Check sheet for the modelled part. Datum: model origin and axes. Units: mm. A direction names the side the tool comes from. Coordinates: 2 decimals unless noted, no trailing zeros. Write each loop counter-clockwise with the first axis right and the second up, starting at its lowest first coordinate (ties: lowest second). Pieces come first, ordered by that corner, then holes. Notation, with made-up numbers: M 72.5,6 L 82.5,6 A23 cw 82.5,18 Z; hole C -33.5,49.25 d4. An arc over 180 degrees is marked long. Answer as CSV lines item,"result". Start each with the question number.
1) Material ranges on L1, parallel to Y at x = 0, z = 1.1; L2, parallel to X at y = 29.5, z = 0.3; L3, parallel to X at y = -2.5, z = 4.75, recorded low to high. Write a range as [from, to].
2) Draft check along Y on faces 1 (the flat face through (-4.5, -43, 1)), 2 (the flat face through (-38, -62, 3)), 3 (the flat face through (68.5, 1, 4)). Enter one of: +Y half, -Y half, draft (parallel to the pull), parting line (faces both ways), or undercut.
3) Access from +Z, -Z, +X, -X, +Y, -Y to the whole of each face (thin tool, end or side, straight path). Record for faces 4 (the flat face through (36, 60, 4)), 5 (the flat face through (20.71, 42.57, 0.99)).
4) Go/stop test with a flat-tipped pin: pin 1 Ø3 at (x, y) = (0, 8) entering from +Z. Record where the tip stops, or that it passes through.
5) Section check A-A (y = 1). Record the cut outline in (x, z).
6) Section check B-B (y = 47.5). State how many separate pieces and enclosed holes the cut face has, and give its area (3 significant figures).
from build123d import *

# Parameters (mm, degrees)
F0_W     = 64
F0_H     = 120
F2_DEPTH = 2
F3_DEPTH = 6
F4_W     = 6
F4_H     = 12
F4_W_2   = 12
F4_H_2   = 6
F5_DEPTH = 2
F7_DEPTH = 2
F8_W     = 9
F8_H     = 40
F8_R     = 1
F9_DEPTH = 2
F10_R    = 1.99999
F11_R    = 1.99999


# Not quite as in the source:
# - a fillet or chamfer is up to 0.001 mm smaller than in the source, because OpenCascade refuses the exact size


with BuildPart() as f2:
    # F0 (on Top) → F2 (new body)
    with BuildSketch(Plane.XY):
        with Locations((-36.5, 0)):
            Rectangle(F0_W, F0_H)
    extrude(amount=F2_DEPTH)

    # F1 (on Top) → F3 (join)
    with BuildSketch(Plane.XY):
        Polygon((-4.5, 60), (-4.5, 62), (-70.5, 62), (-70.5, -62), (-4.5, -62), (-4.5, -60), (-68.5, -60), (-68.5, 60), align=None)
    extrude(amount=F3_DEPTH)

    # F4 (on face) → F5 (join)
    with BuildSketch(Plane.XY.offset(6)):
        with Locations((-67.5, 46)):
            Rectangle(F4_W, F4_H)
        with Locations((-28.5, 59)):
            Rectangle(F4_W_2, F4_H_2)
        with Locations((-67.5, 22)):
            Rectangle(F4_W, F4_H)
        with Locations((-28.5, -59)):
            Rectangle(F4_W_2, F4_H_2)
        with Locations((-67.5, -22)):
            Rectangle(F4_W, F4_H)
        with Locations((-67.5, -46)):
            Rectangle(F4_W, F4_H)
    extrude(amount=-F5_DEPTH)


with BuildPart() as f2b:
    # F0 (on Top) → F2, piece 2 (new body)
    with BuildSketch(Plane.XY):
        with Locations((36.5, 0)):
            Rectangle(F0_W, F0_H)
    extrude(amount=F2_DEPTH)

    # F1 (on Top) → F3, piece 2 (join)
    with BuildSketch(Plane.XY):
        Polygon((70.5, -62), (70.5, 62), (4.5, 62), (4.5, 60), (68.5, 60), (68.5, -60), (4.5, -60), (4.5, -62), align=None)
    extrude(amount=F3_DEPTH)

    # F4 (on face) → F5, piece 2 (join)
    with BuildSketch(Plane.XY.offset(6)):
        with Locations((67.5, 46)):
            Rectangle(F4_W, F4_H)
        with Locations((67.5, -22)):
            Rectangle(F4_W, F4_H)
        with Locations((67.5, -46)):
            Rectangle(F4_W, F4_H)
        with Locations((28.5, 59)):
            Rectangle(F4_W_2, F4_H_2)
        with Locations((67.5, 22)):
            Rectangle(F4_W, F4_H)
        with Locations((28.5, -59)):
            Rectangle(F4_W_2, F4_H_2)
    extrude(amount=-F5_DEPTH)


with BuildPart() as f7_tool:
    # F6 (on face) → F7 (new body)
    with BuildSketch(Plane(origin=(0, 0, 0), x_dir=(1, 0, 0), z_dir=(0, 0, -1))):
        Polygon((-9.5378331968, 57.0000003456), (-63.1068291486, 57.0000003456), (-36.4934644097, 32.0499709028), align=None)
        Polygon((-7.5, 4.8685980187), (-7.5, 54.7983564456), (-34.2993455202, 29.9929844439), align=None)
        Polygon((-9.8931712199, 3), (-36.5065294908, 27.9500233789), (-63.4621541524, 3), align=None)
        Polygon((-65.4999873492, 5.2016438999), (-38.7006483802, 30.0070098378), (-65.5, 55.1314019813), align=None)
        Polygon((-63.4621541524, -3), (-36.5065294908, -27.9500233789), (-9.8931712199, -3), align=None)
        Polygon((-7.5, -4.8685980187), (-34.2993455202, -29.9929844439), (-7.5, -54.7983564456), align=None)
        Polygon((-9.5378331968, -57.0000003456), (-36.4934644097, -32.0499709028), (-63.1068291486, -57.0000003456), align=None)
        Polygon((-65.5, -55.1314019813), (-38.7006483802, -30.0070098378), (-65.4999873492, -5.2016438999), align=None)
        Polygon((7.5, -54.7983564456), (34.2993455202, -29.9929844439), (7.5, -4.8685980187), align=None)
        Polygon((63.1068291486, -57.0000003456), (36.4934644097, -32.0499709028), (9.5378331968, -57.0000003456), align=None)
        Polygon((65.5, -55.1314019813), (65.4999873492, -5.2016438999), (38.7006483802, -30.0070098378), align=None)
        Polygon((36.5065294908, -27.9500233789), (63.4621541524, -3), (9.8931712199, -3), align=None)
        Polygon((63.4621541524, 3), (36.5065294908, 27.9500233789), (9.8931712199, 3), align=None)
        Polygon((7.5, 4.8685980187), (34.2993455202, 29.9929844439), (7.5, 54.7983564456), align=None)
        Polygon((9.5378331968, 57.0000003456), (36.4934644097, 32.0499709028), (63.1068291486, 57.0000003456), align=None)
        Polygon((65.5, 55.1314019813), (38.7006483802, 30.0070098378), (65.4999873492, 5.2016438999), align=None)
    extrude(amount=-F7_DEPTH)


with BuildPart() as f2_1:
    add(f2.part)

    # F7: cut by f7_tool
    add(f7_tool.part, mode=Mode.SUBTRACT)



with BuildPart() as f2b_1:
    add(f2b.part)

    # F7: cut by f7_tool
    add(f7_tool.part, mode=Mode.SUBTRACT)


with BuildPart() as f2_2:
    add(f2_1.part)

    add(f2b_1.part)  # F9 merges F2b
    # F8 (on face) → F9 (join)
    with BuildSketch(Plane(origin=(0, 0, 0), x_dir=(1, 0, 0), z_dir=(0, 0, -1))):
        Rectangle(F8_W, F8_H)
        with Locations((0, -8)):
            Circle(F8_R, mode=Mode.SUBTRACT)
        with Locations((0, 8)):
            Circle(F8_R, mode=Mode.SUBTRACT)
    extrude(amount=-F9_DEPTH)

    # F10 (radius 2 in the source; OpenCascade refuses exactly that, so slightly less here)
    f10_edges = [f2_2.edges().sort_by_distance(p)[0] for p in [
        (28.5, -56, 4),
        (-28.5, -56, 4),
        (64.5, -46, 4),
        (64.5, -22, 4),
        (-64.5, -46, 4),
        (-64.5, -22, 4),
        (64.5, 22, 4),
        (64.5, 46, 4),
        (-28.5, 56, 4),
        (28.5, 56, 4),
        (-64.5, 22, 4),
        (-64.5, 46, 4),
    ]]
    fillet(f10_edges, radius=F10_R)

    # F11 (radius 2 in the source; OpenCascade refuses exactly that, so slightly less here)
    f11_edges = [f2_2.edges().sort_by_distance(p)[0] for p in [
        (28.5, -60, 4),
        (-28.5, -60, 4),
        (-68.5, -46, 4),
        (-68.5, -22, 4),
        (68.5, -46, 4),
        (68.5, -22, 4),
        (68.5, 46, 4),
        (68.5, 22, 4),
        (28.5, 60, 4),
        (-28.5, 60, 4),
        (-68.5, 22, 4),
        (-68.5, 46, 4),
    ]]
    fillet(f11_edges, radius=F11_R)


solid = f2_2.part
Results found:
1,L1,"y = [-20, -9], [-7, 7], [9, 20]"
1,L2,"x = [-70.5, -65.5], [-39.25, -33.77], [-7.5, -4.5], [4.5, 7.5], [33.77, 39.25], [65.5, 70.5]"
1,L3,"x = [-70.5, -68.5], [68.5, 70.5]"
2,face 1,"draft"
2,face 2,"-Y half"
2,face 3,"undercut"
3,face 4,"+Z"
3,face 5,"+Z, -Z"
4,pin 1,"stops at z = 2"
5,outline,"M -70.5,0 L 70.5,0 L 70.5,6 L 68.5,6 L 68.5,2 L -68.5,2 L -68.5,6 L -70.5,6 Z"
6,separate pieces,"8"
6,enclosed holes,"0"
6,area,"99.2 mm2"
